from build123d import *

# Parameters (mm, degrees)
SKETCH1_R           = 8.5
SKETCH1_R_2         = 4
BOSS_EXTRUDE1_DEPTH = 10
FILLET1_R           = 0.5
CHAMFER1_SIZE       = 0.3


with BuildPart() as part:
    # Sketch1 → Boss-Extrude1 (new body)
    with BuildSketch(Plane.XY):
        Circle(SKETCH1_R)
        Circle(SKETCH1_R_2, mode=Mode.SUBTRACT)
    extrude(amount=BOSS_EXTRUDE1_DEPTH)

    # Fillet1
    fillet1_edges = [part.edges().sort_by_distance(p)[0] for p in [
        (-8.5, 0, 0),
        (-8.5, 0, 10),
    ]]
    fillet(fillet1_edges, radius=FILLET1_R)

    # Chamfer1
    chamfer1_edges = [part.edges().sort_by_distance(p)[0] for p in [
        (-4, 0, 0),
        (-4, 0, 10),
    ]]
    chamfer(chamfer1_edges, length=CHAMFER1_SIZE)


solid = part.part
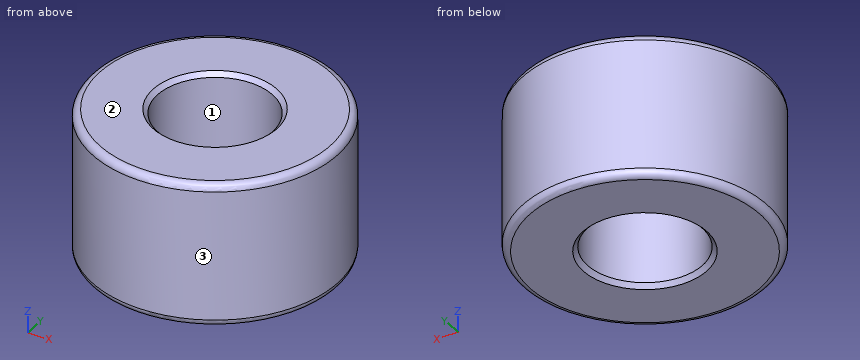
Design review of the part built by this model. Coordinates are the model's own, in mm. Face numbers are marked on the shaded views. Round coordinates to 2 decimals unless told otherwise and drop trailing zeros. Write each loop counter-clockwise with the first axis right and the second up, starting at its lowest first coordinate (ties: lowest second). Pieces come first, ordered by that corner, then holes.
Item 1: For pin 1 Ø1.5 at (y, z) = (4, 7.5) entering from -X; pin 2 Ø1 at (x, z) = (2, 5) entering from +Y; pin 3 Ø6 at (x, z) = (-5.5, 8.5) entering from +Y, all flat-tipped, find the tip position at first contact; note any pin that passes through.
Item 2: Consider section A-A on y = 0. Give the boundary of the cut face in (x, z), and give its area (3 significant figures).
Item 3: Draft analysis for pull direction X (two halves, no side actions). For the marked faces 1, 2 and 3, state which applies: released by +X, released by -X, zero draft, split by the parting line, or undercut.
Item 4: Consider section C-C on z = 1.5. Give the boundary of the cut face in (x, y), and give its area (3 significant figures).
Item 5: Wall thickness on L1, parallel to Y at x = 0, z = 8; L2, parallel to X at y = 7.5, z = 1.75; L3, parallel to Y at x = 1.5, z = 9.5: over which ranges is each line inside the solid? List them lowest first.
Check values:
1. pin 1: stops at x = -7.85
1. pin 2: stops at y = 8.37
1. pin 3: stops at y = 8.12
2. outline: (-8.5, 0.5) arc R0.5 ccw to (-8, 0) - (-4.3, 0) - (-4, 0.3) - (-4, 9.7) - (-4.3, 10) - (-8, 10) arc R0.5 ccw to (-8.5, 9.5) - close; (4, 0.3) - (4.3, 0) - (8, 0) arc R0.5 ccw to (8.5, 0.5) - (8.5, 9.5) arc R0.5 ccw to (8, 10) - (4.3, 10) - (4, 9.7) - close
2. area: 89.6 mm2
3. face 1: undercut
3. face 2: zero draft
3. face 3: split by the parting line
4. outline: circle Ø17 at (0, 0); hole circle Ø8 at (0, 0)
4. area: 177 mm2
5. L1: y = -8.5 to -4, 4 to 8.5
5. L2: x = -4 to 4
5. L3: y = -8.37 to -3.71, 3.71 to 8.37
